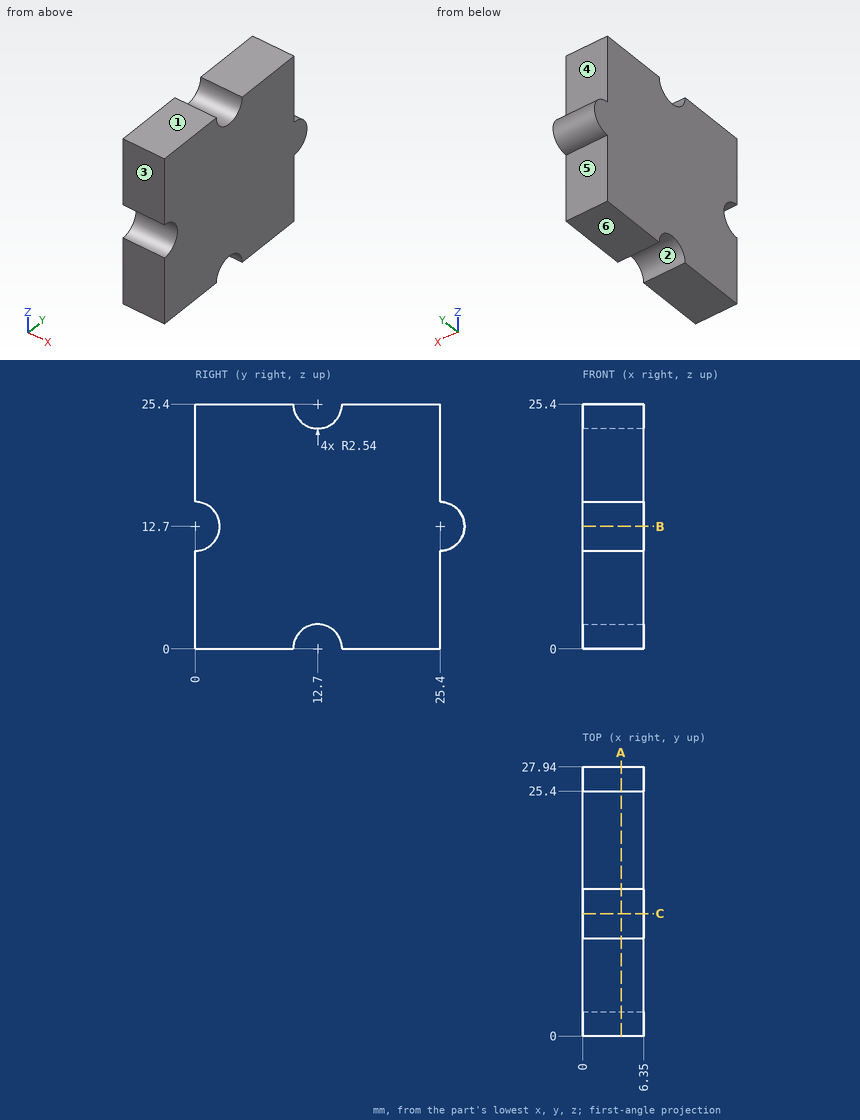
Study the drawing (mm; zero at the part's minimum x, y, z) and answer. A direction names the side the tool comes from. Round coordinates to 2 decimals unless told otherwise and drop trailing zeros. Order: outer loops, then holes, each group sorted by start corner. A loop starts at its lowest first (then second) coordinate and runs counter-clockwise, first axis right, second up. Notation, with made-up numbers: M 39,6 L 73,6 A24 ccw 73,36 Z; hole C 18,-7 d3. An arc over 180 degrees is marked long. One line per item, written item: value.
Q1. Straight lines are drawn through the part: line 1 (Y direction, x = 0.75, z = 21); line 2 (Y direction, x = 3.25, z = 24); line 3 (Y direction, x = 4, z = 23.25). For each, find the intervals that lie inside material, in ascending order.
Derived:
line 1: 0 to 25.4
line 2: 0 to 10.58, 14.82 to 25.4
line 3: 0 to 11.35, 14.05 to 25.4
Q2. Find section A-A on x = 4. Write down the section's boundary in (y, z), then the cut area to 3 significant figures.
Derived:
outline: M 0,0 L 10.16,0 A2.54 cw 15.24,0 L 25.4,0 L 25.4,10.16 A2.54 ccw 25.4,15.24 L 25.4,25.4 L 15.24,25.4 A2.54 cw 10.16,25.4 L 0,25.4 L 0,15.24 A2.54 cw 0,10.16 Z
area: 625 mm²
Q3. Determine the mould class of the marked faces 1, 2 and 3 for opening direction Y: released by +Y, released by -Y, zero draft, split by the parting line, or undercut.
Derived:
face 1: zero draft
face 2: undercut
face 3: released by -Y
Q4. A flat-ended cylindrical pin translates along its axis: pin 1 (1.9 mm diameter, centred on x = 1.5, z = 19.5, fed in from +Y). Find the tip coordinate at first contact, or state that the pin passes through.
Derived:
pin 1: y = 25.4
Q5. For the marked faces 4, 5 and 6, determine the directions among +Z, -Z, +X, -X, +Y, -Y from which every point of the face is accessible in a straight line to the end or side of a thin tool.
Derived:
face 4: +Z, +X, -X, +Y
face 5: -Z, +X, -X, +Y
face 6: -Z, +X, -X, +Y, -Y
Q6. Find section B-B on z = 12.7. Write down the section's boundary in (x, y).
Derived:
outline: M 0,2.54 L 6.35,2.54 L 6.35,27.94 L 0,27.94 Z
Q7. Find section C-C on y = 12.7. Write down the section's boundary in (x, z), then the cut area to 3 significant figures.
Derived:
outline: M 0,2.54 L 6.35,2.54 L 6.35,22.86 L 0,22.86 Z
area: 129 mm²
